Source: CAD feature listing. Evaluate the final solid. Frame: model axes, mm. A direction names the side the tool comes from. Round coordinates to 2 decimals unless told otherwise and drop trailing zeros. Loops run counter-clockwise (first coordinate to the right, second up) from the corner with the lowest first, then second, coordinate; pieces in that order, holes last. Notation, with made-up numbers: (88.25, 6.5) -> (116.25, 6.5) arc R21 ccw to (116.25, 30.5) -> close; hole circle Ø3 at (38, 4). An arc over 180 degrees is marked (long way). Write item = value, one per line.
from build123d import *

# Parameters (mm, degrees)
SKETCH1_W           = 25.4
SKETCH1_H           = 25.4
SKETCH1_W_2         = 22.225
SKETCH1_H_2         = 22.225
BOSS_EXTRUDE1_DEPTH = 501.65
SKETCH4_R           = 6.35
CUT_EXTRUDE1_DEPTH  = 26.4
SKETCH7_R           = 5.08
CUT_EXTRUDE3_DEPTH  = 1.5875


with BuildPart() as part:
    # Sketch1 → Boss-Extrude1 (new body)
    with BuildSketch(Plane(origin=(0, 0, 0), x_dir=(1, 0, 0), z_dir=(0, 1, 0))):
        Rectangle(SKETCH1_W, SKETCH1_H)
        Rectangle(SKETCH1_W_2, SKETCH1_H_2, mode=Mode.SUBTRACT)
    extrude(amount=BOSS_EXTRUDE1_DEPTH)

    # Sketch4 → Cut-Extrude1 (cut, through all)
    with BuildSketch(Plane.XY.offset(12.7)):
        with Locations((0, 9.525)):
            Circle(SKETCH4_R)
    extrude(amount=-CUT_EXTRUDE1_DEPTH, mode=Mode.SUBTRACT)

    # Sketch7 → Cut-Extrude3 (cut)
    with BuildSketch(Plane.XY.offset(12.7)):
        with Locations((0, 63.5)):
            Circle(SKETCH7_R)
    extrude(amount=-CUT_EXTRUDE3_DEPTH, mode=Mode.SUBTRACT)


solid = part.part
1. Section query C-C (y = 384). Return the cut outline in (x, z), then the cut area to 3 significant figures.
Evaluation:
outline = (-12.7, -12.7) -> (12.7, -12.7) -> (12.7, 12.7) -> (-12.7, 12.7) -> close; hole (-11.11, -11.11) -> (11.11, -11.11) -> (11.11, 11.11) -> (-11.11, 11.11) -> close
area = 151 mm²
2. Section query A-A (x = 0). Give the number of separate pieces and of enclosed holes in the cut face, then the cut area to 3 significant figures.
Evaluation:
separate_pieces = 5
enclosed_holes = 0
area = 1,540 mm²
3. Set-up query: faces 1 (the face through (-11.112, 247, 0)), 2 (the face through (2.731, 67.783, 11.917)), 3 (the face through (0, 247, 12.7)). Return all of +Z, -Z, +X, -X, +Y, -Y with unobstructed straight access to the full face (end or side cutting, diameter ignored); none if empty.
Evaluation:
face_1 = +Y, -Y
face_2 = +Z
face_3 = +Z, +X, -X, +Y, -Y
4. Line query: probe 1 along Y at (x, z) = (0, 11.7) (3 decimals); probe 2 along X at (y, z) = (224.5, -8). Output: solid intervals per line, ascending. Write a range as from..to.
Evaluation:
probe_1 = 0..3.175, 15.875..58.42, 68.58..501.65
probe_2 = -12.7..-11.11, 11.11..12.7
5. Section query D-D (y = 63.5). Return the cut outline in (x, z).
Evaluation:
outline = (-12.7, -12.7) -> (12.7, -12.7) -> (12.7, 12.7) -> (5.08, 12.7) -> (5.08, 11.11) -> (11.11, 11.11) -> (11.11, -11.11) -> (-11.11, -11.11) -> (-11.11, 11.11) -> (-5.08, 11.11) -> (-5.08, 12.7) -> (-12.7, 12.7) -> close
6. Section query B-B (z = 1). Return the cut outline in (x, y), then the cut area to 3 significant figures.
Evaluation:
outline = (-12.7, 0) -> (-11.11, 0) -> (-11.11, 501.65) -> (-12.7, 501.65) -> close; (11.11, 0) -> (12.7, 0) -> (12.7, 501.65) -> (11.11, 501.65) -> close
area = 1,590 mm²
7. Mould query, pull axis X, two halves, no side actions, for faces 4 (the face through (0, 247, 11.112)), 5 (the face through (-11.3, 501.65, -0.1)), 6 (the face through (-12.7, 247, 0)). Classes: released by +X, released by -X, zero draft, split by the parting line, or undercut.
Evaluation:
face_4 = undercut
face_5 = zero draft
face_6 = released by -X
8. Contact query for a flat-ended pin moving along its axis: pin 1 Ø6 at (x, z) = (8.5, 0.5) entering from +Y. Output: stop coordinate, or through.
Evaluation:
pin_1 = 501.65
